Input: part model. Units: mm. Frame: model coordinates. A direction names the side the tool comes from. Give positions to 0.01 mm unless a question says otherwise; leave off trailing zeros. Order: outer loops, then holes, each group sorted by start corner. A loop starts at its lowest first (then second) coordinate and runs counter-clockwise, first axis right, second up. Notation, with made-up numbers: (48.25, 4.25) -> (75.25, 4.25) arc R17 cw to (75.25, 35.25) -> close; hole circle Ø5 at (34, -20.5). An arc over 180 degrees is marked (long way). Use a Markdown table: item, result. Add a question column.
from build123d import *

# Parameters (mm, degrees)
ESTRUSIONE_ESTRUSIONE1_DEPTH      = 13
ESTRUSIONE_ESTRUSIONE1_DEPTH_BACK = 3
SCHIZZO1_W                        = 2
SCHIZZO1_H                        = 38.172865154
SCHIZZO2_W                        = 2
SCHIZZO2_H                        = 37
ESTRUSIONE_ESTRUSIONE2_DEPTH      = 5
SCHIZZO3_W                        = 24
SCHIZZO3_H                        = 0.913567423
TAGLIO_ESTRUSIONE1_DEPTH          = 10
RACCORDO1_R                       = 4
RACCORDO1_OF_SPECCHIA1_R          = 4
SCHIZZO4_R                        = 6.5
TAGLIO_ESTRUSIONE2_DEPTH          = 10


with BuildPart() as part:
    # Schizzo1 → Estrusione-Estrusione1 (new, two sides: drawn at the far end of the back side and taken through both)
    with BuildSketch(Plane.XY.offset(-ESTRUSIONE_ESTRUSIONE1_DEPTH_BACK)):
        with Locations((-240, 0)):
            Rectangle(SCHIZZO1_W, SCHIZZO1_H)
    extrude(amount=ESTRUSIONE_ESTRUSIONE1_DEPTH + ESTRUSIONE_ESTRUSIONE1_DEPTH_BACK)

    # Schizzo2 → Estrusione-Estrusione2 (add)
    with BuildSketch(Plane(origin=(0, 19.086432577, 0), x_dir=(1, 0, 0), z_dir=(0, 1, 0))):
        with Locations((-240, -18.5)):
            Rectangle(SCHIZZO2_W, SCHIZZO2_H)
    estrusione_estrusione2 = extrude(amount=ESTRUSIONE_ESTRUSIONE2_DEPTH)

    # Schizzo3 → Taglio-Estrusione1 (cut)
    with BuildSketch(Plane(origin=(-239, 0, 0), x_dir=(0, 0, -1), z_dir=(1, 0, 0))):
        with Locations((-25, 19.543216288)):
            Rectangle(SCHIZZO3_W, SCHIZZO3_H)
    taglio_estrusione1 = extrude(amount=-TAGLIO_ESTRUSIONE1_DEPTH, mode=Mode.SUBTRACT)

    # Raccordo1
    raccordo1_edges = [part.edges().sort_by_distance(p)[0] for p in [
        (-240, 20, 13),
    ]]
    fillet(raccordo1_edges, radius=RACCORDO1_R)

    # Specchia1: Estrusione-Estrusione2, Taglio-Estrusione1 across plane
    add(estrusione_estrusione2.mirror(Plane.ZX))
    add(taglio_estrusione1.mirror(Plane.ZX), mode=Mode.SUBTRACT)

    # Raccordo1 of Specchia1
    raccordo1_of_specchia1_edges = [part.edges().sort_by_distance(p)[0] for p in [
        (-240, -20, 13),
    ]]
    fillet(raccordo1_of_specchia1_edges, radius=RACCORDO1_OF_SPECCHIA1_R)

    # Schizzo4 → Taglio-Estrusione2 (cut)
    with BuildSketch(Plane(origin=(-239, 0, 0), x_dir=(0, 0, -1), z_dir=(1, 0, 0))):
        with Locations((-6, 0)):
            Circle(SCHIZZO4_R)
    extrude(amount=-TAGLIO_ESTRUSIONE2_DEPTH, mode=Mode.SUBTRACT)


solid = part.part
Q1. Ray query, line 1 (Y direction, x = -240.6, z = 6); line 2 (Y direction, x = -239.7, z = 29); line 3 (Z direction, x = -240.9, y = 15.5). Return the intervals inside material, ascending.
Q2. Access query for faces 1 (the cylindrical face through (-240.014, -18.797, 14.141)), 2 (the flat face through (-240, -19.086, -2)), 3 (the flat face through (-240, 19.086, -2)), 4 (the flat face through (-240, 24.086, 18)). Directions: +Z, -Z, +X, -X, +Y, -Y. A direction counts if a zero-diameter tool reaches every point of the face in a straight line with its end or side. Return the directions, or none.
Q3. Draft query along Y for faces 5 (the cylindrical face through (-240.014, 18.797, 14.141)), 6 (the flat face through (-240, -22, 0)), 7 (the cylindrical face through (-239.99, 1.95, -0.2)), 8 (the flat face through (-240, -24.086, 18)). Return one class per face: +Y half, -Y half, draft (parallel to the pull), parting line (faces both ways), or undercut.
Q4. Section query D-D (y = -12). Return loops of the section in (x, z).
Q5. Section query C-C (x = -240.35). Return loops of the section in (y, z).
Q6. Section query A-A (z = 21.5). Return loops of the section in (x, y).
Q7. Section query B-B (y = 0). Return loops of the section in (x, z), plus the area to 3 significant figures.
Q8. First-contact query: pin 1 (1 mm diameter, centred on x = -239.5, y = -2.5, fed in from +Z). Flat tip, straight axial feed; report the tip coordinate or a pass-through.
Solution:
| question | item | result |
|---|---|---|
| 1 | line 1 | y = -24.09 to -6.5, 6.5 to 24.09 |
| 1 | line 2 | y = -24.09 to -20, 20 to 24.09 |
| 1 | line 3 | z = -3 to 13 |
| 2 | face 1 | +Z, +X, -X |
| 2 | face 2 | -Z, +X, -X, -Y |
| 2 | face 3 | -Z, +X, -X, +Y |
| 2 | face 4 | +Z, -Z, +X, -X, +Y |
| 3 | face 5 | undercut |
| 3 | face 6 | draft |
| 3 | face 7 | undercut |
| 3 | face 8 | -Y half |
| 4 | outline | (-241, -3) -> (-239, -3) -> (-239, 13) -> (-241, 13) -> close |
| 5 | outline | (-24.09, 0) -> (-19.09, 0) -> (-19.09, -3) -> (19.09, -3) -> (19.09, 0) -> (24.09, 0) -> (24.09, 37) -> (20, 37) -> (20, 17) arc R4 cw to (16, 13) -> (-16, 13) arc R4 cw to (-20, 17) -> (-20, 37) -> (-24.09, 37) -> close; hole circle Ø13 at (0, 6) |
| 6 | outline | (-241, -24.09) -> (-239, -24.09) -> (-239, -20) -> (-241, -20) -> close; (-241, 20) -> (-239, 20) -> (-239, 24.09) -> (-241, 24.09) -> close |
| 7 | outline | (-241, -3) -> (-239, -3) -> (-239, -0.5) -> (-241, -0.5) -> close; (-241, 12.5) -> (-239, 12.5) -> (-239, 13) -> (-241, 13) -> close |
| 7 | area | 6.00 mm² |
| 8 | pin 1 | stops at z = 13 |
